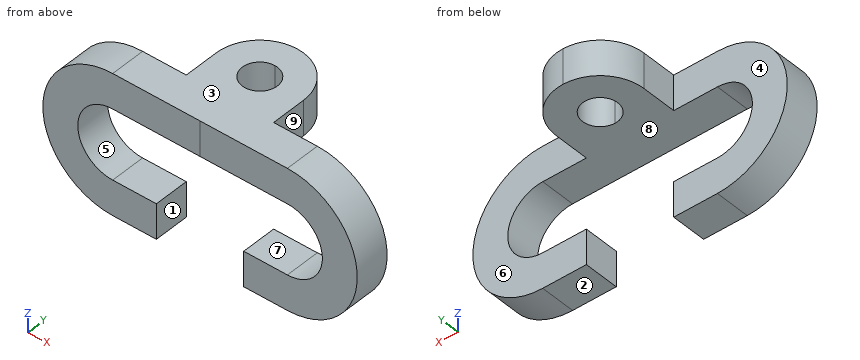
from build123d import *

# Parameters (mm, degrees)
F1_DEPTH = 12.7
F3_DEPTH = 12.7


with BuildPart() as f1:
    # F0 (on Front) → F1 (new body)
    with BuildSketch(Plane.XZ):
        with BuildLine():
            Line((31.75, 0), (0, 0))
            Line((0, 0), (0, -12.7))
            Line((0, -12.7), (31.75, -12.7))
            ThreePointArc((31.75, -12.7), (44.45, -25.4), (31.75, -38.1))
            Line((31.75, -38.1), (15.875, -38.1))
            Line((15.875, -38.1), (15.875, -50.8))
            Line((15.875, -50.8), (31.75, -50.8))
            ThreePointArc((31.75, -50.8), (57.15, -25.4), (31.75, 0))
        make_face()
    extrude(amount=F1_DEPTH)

    # F2 (on face) → F3 (join, through all)
    with BuildSketch(Plane.XY):
        with BuildLine():
            Line((15.875, 0), (15.875, 12.7))
            ThreePointArc((15.875, 12.7), (11.22532, 23.92532), (0, 28.575))
            Line((0, 28.575), (0, 19.05))
            ThreePointArc((0, 19.05), (6.35, 12.7), (0, 6.35))
            Line((0, 6.35), (0, 0))
            Line((0, 0), (15.875, 0))
        make_face()
    extrude(amount=-F3_DEPTH)

    # F4: F1 across face


with BuildPart() as f1_1:
    add(f1.part)
    add(f1.part.mirror(Plane(origin=(0, -3.175, -6.35), x_dir=(0, -1, 0), z_dir=(-1, 0, 0))))


solid = f1_1.part
Check sheet for the modelled part. Datum: model origin and axes. Units: mm. Face numbers are marked on the shaded views. A direction names the side the tool comes from. Round coordinates to 2 decimals unless told otherwise and drop trailing zeros. Order: outer loops, then holes, each group sorted by start corner. A loop starts at its lowest first (then second) coordinate and runs counter-clockwise, first axis right, second up.
Q1. Cross-section at A-A, the plane x = 26.5. Enter the section's corners in (y, z).
Filled sheet:
outline: (-12.7, -50.8) - (0, -50.8) - (0, -38.1) - (-12.7, -38.1) - close; (-12.7, -12.7) - (0, -12.7) - (0, 0) - (-12.7, 0) - close
Q2. Cross-section at B-B, the plane z = -25.4. Enter the section's corners in (x, y).
Filled sheet:
outline: (-57.15, -12.7) - (-44.45, -12.7) - (-44.45, 0) - (-57.15, 0) - close; (44.45, -12.7) - (57.15, -12.7) - (57.15, 0) - (44.45, 0) - close
Q3. Cross-section at D-D, the plane z = -3.5. Enter the section's corners in (x, y) (3 decimals), plus the area to 3 significant figures.
Filled sheet:
outline: (-44.617, -12.7) - (44.617, -12.7) - (44.617, 0) - (15.875, 0) - (15.875, 12.7) arc R15.875 ccw to (0, 28.575) arc R15.875 ccw to (-15.875, 12.7) - (-15.875, 0) - (-44.617, 0) - close; hole circle Ø12.7 at (0, 12.7)
area: 1,810 mm2
Q4. Depth check by flat-ended pin: P1, Ø8, axis at y = 19.5, z = -10, coming from the -X side; P2, Ø20.5, axis at x = 10, y = 9.5, coming from the -Z side; P3, Ø14, axis at y = -4.5, z = -46, coming from the -X side. Enter the tip coordinate at first touch or a pass-through.
Filled sheet:
P1: stops at x = -15.63
P2: stops at z = -12.7
P3: stops at x = -53.2
Q5. Draft check along X on the marked faces 6, 7, 8 and 9. Enter one of: pulls with the +X half, pulls with the -X half, needs draft (parallel to the pull), parting line crosses it, or undercut.
Filled sheet:
face 6: needs draft
face 7: undercut
face 8: undercut
face 9: pulls with the +X half
Q6. Scan lines: L1, parallel to Z at x = 6, y = 0; L2, parallel to X at y = 14.5, z = -3.5. Record each from-to range of solid material in increasing order.
Filled sheet:
L1: z = -12.7 to 0
L2: x = -15.77 to -6.09, 6.09 to 15.77
Q7. Cross-section at C-C, the plane y = -7.5. Enter the section's corners in (x, z) (3 decimals).
Filled sheet:
outline: (-31.75, -50.8) - (-15.875, -50.8) - (-15.875, -38.1) - (-31.75, -38.1) arc R12.7 cw to (-31.75, -12.7) - (31.75, -12.7) arc R12.7 cw to (31.75, -38.1) - (15.875, -38.1) - (15.875, -50.8) - (31.75, -50.8) arc R25.4 ccw to (31.75, 0) - (-31.75, 0) arc R25.4 ccw to start
Q8. Set-up check for the marked faces 1, 2, 3, 4 and 5: record each of +Z, -Z, +X, -X, +Y, -Y from which the full face is reachable in a straight line by a thin tool's end or side.
Filled sheet:
face 1: -Z, +Y, -Y
face 2: -Z, +X, -X, +Y, -Y
face 3: +Z, +X, -X, +Y, -Y
face 4: +Z, -Z, -X, +Y
face 5: +Y, -Y
